Read the model definition and answer for the solid it produces. Units are mm, in the model's axes. A direction names the side the tool comes from. Round coordinates to 2 decimals unless told otherwise and drop trailing zeros. Write each loop counter-clockwise with the first axis right and the second up, starting at its lowest first coordinate (ties: lowest second). Pieces come first, ordered by that corner, then holes. Notation, with made-up numbers: (42, -35) -> (85, -35) arc R15 cw to (85, -17) -> close; hole circle Ø3 at (-29.5, -17.5). An arc over 180 degrees is marked (long way). Return JSON: item names as keys, results as strings.
Autodesk Inventor part; units mm, degrees
ref_plane "YZ Plane" through (0, 0, 0) normal (1, 0, 0) x (0, 1, 0)
ref_plane "XZ Plane" through (0, 0, 0) normal (0, 1, 0) x (-1, 0, 0)
ref_plane "XY Plane" through (0, 0, 0) normal (0, 0, 1) x (1, 0, 0)
sketch "Sketch1" plane through (0, 0, 0) normal (0, 1, 0) x (-1, 0, 0)
  circle A0 centre (-26.1551, -3.0475) radius 2
  arc A1 (-34.9051, -0.0475) -> (-17.4051, -0.0475) centre (-26.1551, -0.0475) ccw
  arc A2 (17.5949, -0.0475) -> (35.0949, -0.0475) centre (26.3449, -0.0475) ccw
  circle A3 centre (26.3449, -3.0475) radius 2
  circle A4 centre (-26.1551, -3.0475) radius 2
  circle A5 centre (26.3449, -3.0475) radius 2
  circle A6 centre (26.3449, -0.0475) radius 8.75
  circle A7 centre (-26.1551, -0.0475) radius 8.75
  line L0 (-34.9051, -0.0475) -> (-17.4051, -0.0475)
  line L1 (17.5949, -0.0475) -> (35.0949, -0.0475)
  circle A8 centre (-26.1551, -3.0475) radius 5.5
  circle A9 centre (26.3449, -3.0475) radius 5.5
  line L2 (-26.1551, -8.5475) -> (26.3449, -8.5475)
  line L3 (-26.1551, 2.4525) -> (26.3449, 2.4525)
  point P0 (0, 0)
  dimension "d0" = 11
  dimension "d1" = 11
extrude "Extrusion1" add sketch "Sketch1" along normal blind 10 contours L2 A8 L0 A1 | A1 A7 L3 A6 A2 L2 | A7 L0 A8 L3 | A8 L0 | L0 A8 | A2 L1 A9 L2 | L3 A9 L1 A6 | A9 L1 | A9 L1 picked at (-18.6939, -1.0014) picked at (-20.5799, 1.133) picked at (18.8536, -1.0809) picked at (20.7697, 1.133)
sketch "Sketch2" plane through (0, 10, 0) normal (0, 1, 0) x (1, 0, 0)
  line L0 (26.1551, 8.5475) -> (-26.3449, 8.5475)
  line L1 (-26.3449, -2.4525) -> (26.1551, -2.4525)
  arc A0 (-26.3449, 8.5475) -> (-26.3449, -2.4525) centre (-26.3449, 3.0475) ccw
  arc A1 (26.1551, -2.4525) -> (26.1551, 8.5475) centre (26.1551, 3.0475) ccw
  line L2 (-31.8449, 3.0475) -> (31.6551, 3.0475)
  line L3 (13.4051, -3.4525) -> (-13.5949, -3.4525)
  line L4 (-13.5949, -3.4525) -> (-13.5949, 9.5475)
  line L5 (-13.5949, 9.5475) -> (13.4051, 9.5475)
  line L6 (13.4051, 9.5475) -> (13.4051, -3.4525)
  line L7 (13.4051, -3.4525) -> (-13.5949, 9.5475) construction
  line L8 (-13.5949, -3.4525) -> (13.4051, 9.5475) construction
  point P0 (0, 0)
  point P1 (-0.0949, 3.0475)
  dimension "d4" = 27
  dimension "d5" = 13
extrude "Extrusion2" add sketch "Sketch2" along normal blind 14.56 contours L6 L2 L4 L0 | L0 L4 L5 L6 | L6 L1 L4 L2 | L6 L3 L4 L1
fillet "Fillet1" radius 2 2 edges at (-0.0949, 10, 3.4525) (-0.0949, 10, -9.5475)
sketch "Sketch3" plane through (0, 24.56, 0) normal (0, 1, 0) x (1, 0, 0)
  arc A0 (-6.3236, 1.0357) -> (-4.0158, 1.1475) centre (-5.0949, -0.4525) ccw
  arc A1 (3.5842, 1.1475) -> (6.0652, 1.2676) centre (4.9051, -0.4525) ccw
  circle A2 centre (4.9051, -0.4525) radius 2.0748
  circle A3 centre (-5.0949, -0.4525) radius 1.9299
  line L0 (-13.5949, 9.5475) -> (-13.5949, -3.4525)
  line L1 (13.4051, 9.5475) -> (-13.5949, 9.5475)
  line L2 (-13.5949, -3.4525) -> (13.4051, -3.4525)
  line L3 (13.4051, -3.4525) -> (13.4051, 9.5475)
  point P0 (0, 0)
  point P1 (6.0652, 1.2676)
  point P2 (-4.0158, 1.1475)
  dimension "d12" = 8.5
  dimension "d13" = 8.5
extrude "Extrusion3" cut sketch "Sketch3" against normal blind 10 contours A3 A0 | A2 A1
sketch "Sketch4" plane through (0, 24.56, 0) normal (0, 1, 0) x (1, 0, 0)
  line L0 (13.4051, 9.5475) -> (-13.5949, 9.5475)
  line L1 (-13.5949, -2.4525) -> (-13.5949, 8.5475)
  line L2 (13.4051, 9.5475) -> (-13.5949, 9.5475)
  line L3 (-13.5949, 9.5475) -> (-13.5949, 3.0475)
  line L4 (-13.5949, 3.0475) -> (13.4051, 3.0475)
  line L5 (13.4051, 3.0475) -> (13.4051, 9.5475)
  point P0 (0, 0)
extrude "Extrusion4" cut sketch "Sketch4" against normal blind 4.2875
fillet "Fillet2" radius 6.7625 1 edges at (-0.0949, 20.2725, -9.5475)
sketch "Sketch5" plane through (0, 24.56, 0) normal (0, 1, 0) x (1, 0, 0)
  line L0 (-13.5949, 3.0475) -> (-13.5949, 9.5475)
  line L1 (13.4051, -3.4525) -> (-13.5949, -3.4525)
  line L2 (-13.5949, 3.0475) -> (13.4051, 3.0475)
  line L3 (13.4051, 3.0475) -> (13.4051, -3.4525)
  line L4 (13.4051, -3.4525) -> (-13.5949, -3.4525)
  line L5 (-13.5949, -3.4525) -> (-13.5949, 3.0475)
  line L6 (0.5551, -10.9283) -> (-0.7449, -10.9283)
  line L7 (-0.7449, -10.9283) -> (-0.7449, 4.0233)
  line L8 (-0.7449, 4.0233) -> (0.5551, 4.0233)
  line L9 (0.5551, 4.0233) -> (0.5551, -10.9283)
  line L10 (0.5551, -10.9283) -> (-0.7449, 4.0233) construction
  line L11 (-0.7449, -10.9283) -> (0.5551, 4.0233) construction
  point P0 (0, 0)
  point P1 (-0.0949, -3.4525)
  dimension "d19" = 1.3
extrude "Extrusion5" cut sketch "Sketch5" against normal blind 6 contours L9 L6 L7 L1 | L1 L7 L2 L9 | L2 L7 L8 L9
properties part number "Servo Holder short side"
Item 1: A tool of negligible diameter and unlimited length cuts with its end or side. For faces 1 (the flat face through (0, 5, 2.452)), 2 (the flat face through (0, 18.56, 0)), 3 (the flat face through (-5, 14.56, 0)), 4 (the flat face through (23, 10, -3)), 5 (the flat face through (-13.595, 16, -2)), from which of +Z, -Z, +X, -X, +Y, -Y can it reach the whole face along a straight path? Write none if from no direction.
Worked answers:
{"face 1": "+Z, +X, -X, -Y", "face 2": "+Z, +Y", "face 3": "+Y", "face 4": "+Z, -Z, +X, +Y", "face 5": "+Z, -Z, -X, +Y"}
Item 2: Section D-D (x = 9.5) is taken. Give the vertices of the cut face in (y, z) (1 decimal), then the cut area to 3 significant figures.
Worked answers:
{"outline": "(0, -8.5) -> (10, -8.5) arc R2 ccw to (11.7, -9.5) -> (13.5, -9.5) arc R6.8 ccw to (20.3, -3) -> (24.6, -3) -> (24.6, 3.5) -> (11.7, 3.5) arc R2 ccw to (10, 2.5) -> (0, 2.5) -> close", "area": "261 mm2"}
Item 3: Section C-C (z = -2.25) is taken. Give the vertices of the cut face in (x, y), then the cut area to 3 significant figures.
Worked answers:
{"outline": "(-31.79, 0) -> (-28.18, 0) -> (-28.18, 10) -> (-31.79, 10) -> close; (-24.51, 0) -> (24.32, 0) -> (24.32, 10) -> (13.41, 10) -> (13.41, 24.56) -> (0.56, 24.56) -> (0.56, 18.56) -> (-0.74, 18.56) -> (-0.74, 24.56) -> (-13.59, 24.56) -> (-13.59, 10) -> (-24.51, 10) -> close; (27.99, 0) -> (31.6, 0) -> (31.6, 10) -> (27.99, 10) -> close", "area": "946 mm2"}
Item 4: Straight lines are drawn through the part: L1, parallel to X at y = 3.25, z = -2.5; L2, parallel to X at y = 2, z = -2; L3, parallel to Y at x = 26.5, z = -1. For each, find the intervals that lie inside material, in ascending order. Write a range as [from, to].
Worked answers:
{"L1": "x = [-31.82, -28.27], [-24.42, 24.23], [28.08, 31.63]", "L2": "x = [-31.74, -28.05], [-24.64, 24.45], [27.86, 31.55]", "L3": "y = [0, 10]"}
Item 5: Flat-ended cylindrical pins translate along their axes: pin 1 (1.5 mm diameter, centred on y = 8, z = -5, fed in from +X); pin 2 (5 mm diameter, centred on x = -6, y = 3, fed in from -Z); pin 3 (1 mm diameter, centred on x = -17, y = 6, fed in from +Z). Find the tip coordinate at first contact, or state that the pin passes through.
Worked answers:
{"pin 1": "stops at x = 31.52", "pin 2": "stops at z = -8.55", "pin 3": "stops at z = 2.45"}
Item 6: Section A-A (x = -27) is taken. Give the vertices of the cut face in (y, z), then the cut area to 3 significant figures.
Worked answers:
{"outline": "(0, -8.51) -> (10, -8.51) -> (10, -4.94) -> (0, -4.94) -> close; (0, -1.16) -> (10, -1.16) -> (10, 2.41) -> (0, 2.41) -> close", "area": "71.4 mm2"}
Item 7: For a pull along Z with two mould halves and no side action, classify faces 6 (the cylindrical face through (-28.25, 4.93, -3.65)), 7 (the flat face through (0, 18, 3.452)), 8 (the flat face through (0, 5, -8.548)), 9 (the flat face through (-7.3, 24.56, 0.2)) as released by +Z, released by -Z, zero draft, split by the parting line, or undercut.
Worked answers:
{"face 6": "undercut", "face 7": "released by +Z", "face 8": "released by -Z", "face 9": "zero draft"}
Item 8: Section B-B (y = 8.75) is taken. Give the vertices of the cut face in (x, z), then the cut area to 3 significant figures.
Worked answers:
{"outline": "(-26.34, -8.55) -> (26.16, -8.55) arc R5.5 ccw to (26.16, 2.45) -> (-26.34, 2.45) arc R5.5 ccw to start; hole circle Ø4 at (-26.34, -3.05); hole circle Ø4 at (26.16, -3.05)", "area": "647 mm2"}
